Verification items for this drawing (mm, ordinates from the low corner). Round coordinates to 2 decimals unless told otherwise and drop trailing zeros. Loops run counter-clockwise (first coordinate to the right, second up) from the corner with the lowest first, then second, coordinate; pieces in that order, holes last. Notation, with made-up numbers: (-27.5, 85.25) -> (1.5, 85.25) arc R10 cw to (1.5, 102.25) -> close; hole circle Ø9 at (62, 67.25). An arc over 180 degrees is marked (long way). Use a Markdown table: item, result. Add a question column.
Q1. Sectioned sample at A-A, the plane x = 9.25. Enter the section's corners in (y, z).
Q2. Sectioned sample at C-C, the plane z = 6.5. Enter the section's corners in (x, y).
Q3. Material ranges on L1, parallel to Z at x = 33.25, y = 1.65; L2, parallel to X at y = 1.75, z = 8.25; L3, parallel to X at y = 1.4, z = 9.5, recorded low to high.
Q4. Sectioned sample at B-B, the plane y = 1.1. Enter the section's corners in (x, z), then the cut area to 3 significant figures.
Q5. Gauge pin test, flat end, axial feed: P1, Ø5.5, axis at x = 9.25, z = 6.5, coming from the -Y side. Record the tip position at first contact, or that the pin passes through.
Q6. Sectioned sample at D-D, the plane x = 33.25. Enter the section's corners in (y, z), then the cut area to 3 significant figures.
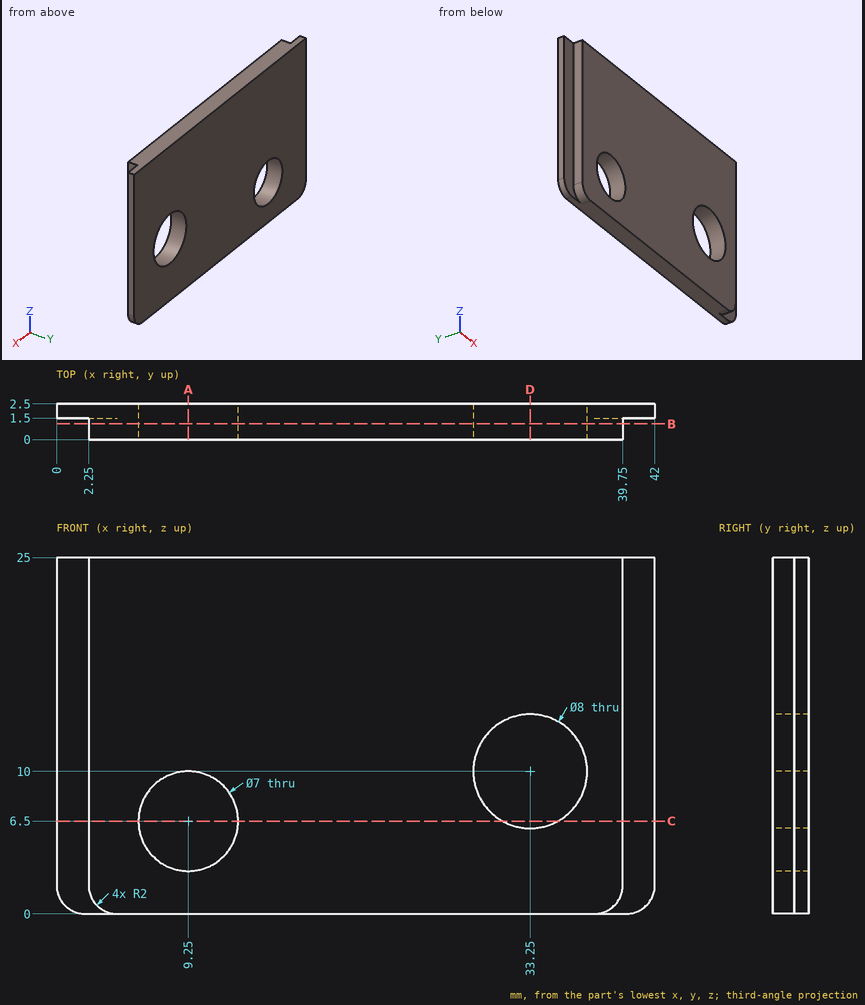
Values:
| question | item | result |
|---|---|---|
| 1 | outline | (0, 0) -> (2.5, 0) -> (2.5, 3) -> (0, 3) -> close; (0, 10) -> (2.5, 10) -> (2.5, 25) -> (0, 25) -> close |
| 2 | outline | (0, 1.5) -> (2.25, 1.5) -> (2.25, 0) -> (5.75, 0) -> (5.75, 2.5) -> (0, 2.5) -> close; (12.75, 0) -> (31.31, 0) -> (31.31, 2.5) -> (12.75, 2.5) -> close; (35.19, 0) -> (39.75, 0) -> (39.75, 1.5) -> (42, 1.5) -> (42, 2.5) -> (35.19, 2.5) -> close |
| 3 | L1 | 0 to 6, 14 to 25 |
| 3 | L2 | 0 to 6.22, 12.28 to 29.65, 36.85 to 42 |
| 3 | L3 | 2.25 to 7.45, 11.05 to 29.28, 37.22 to 39.75 |
| 4 | outline | (2.25, 2) arc R2 ccw to (4.25, 0) -> (37.75, 0) arc R2 ccw to (39.75, 2) -> (39.75, 25) -> (2.25, 25) -> close; hole circle Ø7 at (9.25, 6.5); hole circle Ø8 at (33.25, 10) |
| 4 | area | 847 mm^2 |
| 5 | P1 | through |
| 6 | outline | (0, 0) -> (2.5, 0) -> (2.5, 6) -> (0, 6) -> close; (0, 14) -> (2.5, 14) -> (2.5, 25) -> (0, 25) -> close |
| 6 | area | 42.5 mm^2 |
